Autodesk Inventor part; units mm, degrees
ref_plane "YZ Plane" through (0, 0, 0) normal (1, 0, 0) x (0, 1, 0)
ref_plane "XZ Plane" through (0, 0, 0) normal (0, 1, 0) x (-1, 0, 0)
ref_plane "XY Plane" through (0, 0, 0) normal (0, 0, 1) x (1, 0, 0)
sketch "Szkic1" plane through (0, 0, 0) normal (0, 0, 1) x (1, 0, 0)
  line L0 (-13.054, 5.3954) -> (8.946, 5.3954)
  line L1 (8.946, 5.3954) -> (8.946, -6.6046)
  line L2 (8.946, -6.6046) -> (-13.054, -6.6046)
  line L3 (-13.054, -6.6046) -> (-13.054, 5.3954)
  point P0 (0, 0)
  dimension "d0" = 22
  dimension "d1" = 12
extrude "Wyciągnięcie proste1" add sketch "Szkic1" along normal blind 12.7
fillet "Zaokrąglenie1" radius 2.5 2 edges at (-13.054, 5.3954, 6.35) (8.946, 5.3954, 6.35)
sketch "Szkic2" plane through (0, 0, 12.7) normal (0, 0, 1) x (1, 0, 0)
  line L0 (8.946, -6.6046) -> (8.946, 2.8954)
  line L1 (-13.054, 2.8954) -> (-13.054, -6.6046)
  circle A0 centre (-2.054, -6.8046) radius 8.075
  line L2 (6.446, 5.3954) -> (-10.554, 5.3954)
  point P0 (0, 0)
  dimension "d5" = 22
  dimension "d6" = 11
  dimension "d7" = 16.15
  dimension "d10" = 12.2
extrude "Wyciągnięcie proste2" cut sketch "Szkic2" against normal blind 12.7
sketch "Szkic3" plane through (0, 0, 12.7) normal (0, 0, 1) x (1, 0, 0)
  arc A0 (6.0185, -6.6046) -> (-10.1265, -6.6046) centre (-2.054, -6.8046) ccw
  line L0 (6.0185, -6.6046) -> (8.946, -6.6046)
  line L1 (8.946, -6.6046) -> (8.946, 2.8954)
  arc A1 (8.946, 2.8954) -> (6.446, 5.3954) centre (6.446, 2.8954) ccw
  line L2 (6.446, 5.3954) -> (-10.554, 5.3954)
  arc A2 (-10.554, 5.3954) -> (-13.054, 2.8954) centre (-10.554, 2.8954) ccw
  line L3 (-13.054, 2.8954) -> (-13.054, -6.6046)
  line L4 (-13.054, -6.6046) -> (-10.1265, -6.6046)
  arc A3 (3.9927, -6.6046) -> (-8.1007, -6.6046) centre (-2.054, -6.8046) ccw
  arc A4 (6.0185, -6.6046) -> (-10.1265, -6.6046) centre (-2.054, -6.8046) ccw
  line L5 (6.0185, -6.6046) -> (-10.1265, -6.6046)
  point P0 (0, 0)
  dimension "d11" = 12.1
extrude "Wyciągnięcie proste3" add sketch "Szkic3" against normal blind 8.55 contours L5 A3 A0
extrude "Wyciągnięcie proste4" cut sketch "Szkic3" against normal blind 3.45 contours L5 A3 A0
sketch "Szkic4" plane through (-13.054, -6.6046, 0) normal (0, -1, 0) x (1, 0, 0)
  line L0 (0, 0) -> (0, 12.7)
  line L1 (22, 0) -> (22, 12.7)
  line L2 (4.9533, 9.25) -> (2.9275, 9.25)
  line L3 (19.0725, 9.25) -> (17.0467, 9.25)
  line L4 (4.9533, 9.25) -> (4.9533, 4.15)
  line L5 (4.9533, 4.15) -> (2.9275, 4.15)
  point P0 (13.054, 0)
  point P1 (2.4767, 6.7)
  point P2 (19.5233, 6.7)
  dimension "d16" = 2.4766
  dimension "d17" = 2.4766
  dimension "d18" = 2.55
  dimension "d19" = 2.55
  dimension "d33" = 4.9533
  dimension "d34" = 5.1
hole "Otwór1" at (-10.5773, -6.6046, 6.7) at (6.4694, -6.6046, 6.7) direction (0, 1, 0) diameter 3.2 end through all
sketch "Szkic5" plane through (-10.554, 5.3954, 0) normal (0, 1, 0) x (1, 0, 0)
  arc A0 (0, -8.2998) -> (0, -5.1002) centre (-0.0233, -6.7) ccw
  line L0 (0, -12.7) -> (0, -8.2998)
  line L1 (17, -12.7) -> (0, -12.7)
  line L2 (17, -8.2998) -> (17, -12.7)
  arc A1 (17, -5.1002) -> (17, -8.2998) centre (17.0233, -6.7) ccw
  line L3 (17, 0) -> (17, -5.1002)
  line L4 (0, 0) -> (17, 0)
  line L5 (0, -5.1002) -> (0, 0)
  line L6 (19.5, -12.7) -> (19.5, 0)
  line L7 (-2.5, 0) -> (-2.5, -12.7)
  line L8 (-3.125, -4.9102) -> (-0.025, -3.1204)
  line L9 (-0.025, -3.1204) -> (3.075, -4.9102)
  line L10 (3.075, -4.9102) -> (3.075, -8.4898)
  line L11 (3.075, -8.4898) -> (-0.025, -10.2796)
  line L12 (-0.025, -10.2796) -> (-3.125, -8.4898)
  line L13 (-3.125, -8.4898) -> (-3.125, -4.9102)
  line L14 (13.9, -4.9102) -> (17, -3.1204)
  line L15 (17, -3.1204) -> (20.1, -4.9102)
  line L16 (20.1, -4.9102) -> (20.1, -8.4898)
  line L17 (20.1, -8.4898) -> (17, -10.2796)
  line L18 (17, -10.2796) -> (13.9, -8.4898)
  line L19 (13.9, -8.4898) -> (13.9, -4.9102)
  point P0 (10.554, 0)
  point P1 (17, -6.7)
  point P2 (-0.025, -6.7)
  point P3 (-0.025, -6.7)
  point P4 (-3.125, -6.7)
  point P5 (17, -6.7)
  point P6 (13.9, -6.7)
extrude "Wyciągnięcie proste6" cut sketch "Szkic5" against normal blind 4 contours L0 L11 L12 L7 L8 L9 L5 A0 | A0 L5 L9 L10 L11 L0 | L12 L13 L8 L7 | L18 L19 L14 L3 A1 L2 | L2 A1 L3 L15 L6 L17 | L6 L15 L16 L17
properties part number "3DP_ABS_E3DV6_Mounting_Clamp"
Here's how the part is built. I have some questions about the finished solid (model axes, mm). A direction names the side the tool comes from. Give positions to 0.01 mm unless a question says otherwise; leave off trailing zeros. Loops run counter-clockwise (first coordinate to the right, second up) from the corner with the lowest first, then second, coordinate; pieces in that order, holes last. Notation, with made-up numbers: M -4.5,16.5 L 51.5,16.5 A25 ccw 51.5,35.5 Z; hole C 43,68.5 d8. An arc over 180 degrees is marked long. Return JSON: item names as keys, results as strings.
Item 1: Imagine slicing it at D-D on y = 2.5. List the corners of the cut face in (x, z) for me.
A:
{"outline": "M -13.05,0 L 8.95,0 L 8.95,4.56 L 6.45,3.12 L 3.35,4.91 L 3.35,8.49 L 6.45,10.28 L 8.95,8.84 L 8.95,12.7 L -13.05,12.7 L -13.05,8.85 L -10.58,10.28 L -7.48,8.49 L -7.48,4.91 L -10.58,3.12 L -13.05,4.55 Z"}
Item 2: I'm going to push flat-ended pins straight in: pin 1 Ø6 at (x, z) = (7, 7) entering from +Y; pin 2 Ø1.5 at (x, y) = (3, -4.5) entering from -Z; pin 3 Ø5 at (y, z) = (3, 6) entering from +X; pin 4 Ø1.1 at (y, z) = (3, 7) entering from +X. Where does each tip first touch, or does it pass through?
A:
{"pin 1": "stops at y = 5.35", "pin 2": "stops at z = 4.15", "pin 3": "stops at x = 8.95", "pin 4": "stops at x = 3.35"}
Item 3: Please list where these lines run through material, in increasing order: line 1 (X direction, y = -3, z = 6.7); line 2 (X direction, y = -3.75, z = 6.7); line 3 (X direction, y = -3.75, z = 9.5).
A:
{"line 1": "x = -13.05 to -12.18, -8.98 to -6.76, 2.65 to 4.87, 8.07 to 8.95", "line 2": "x = -13.05 to -12.18, -8.98 to -7.28, 3.17 to 4.87, 8.07 to 8.95", "line 3": "x = -13.05 to -9.53, 5.42 to 8.95"}
Item 4: Imagine slicing it at A-A on z = 6.7. List the corners of the cut face in (x, y) for me.
A:
{"outline": "M -13.05,-6.6 L -12.18,-6.6 L -12.18,1.4 L -13.05,1.4 Z; M -8.98,-6.6 L -8.1,-6.6 A6.05 cw 3.99,-6.6 L 4.87,-6.6 L 4.87,1.4 L 3.35,1.4 L 3.35,5.4 L -7.48,5.4 L -7.48,1.4 L -8.98,1.4 Z; M 8.07,-6.6 L 8.95,-6.6 L 8.95,1.4 L 8.07,1.4 Z"}
Item 5: Imagine slicing it at C-C on x = 7. List the corners of the cut face in (y, z) for me, then the cut area to 3 significant figures.
A:
{"outline": "M -6.6,0 L 5.33,0 L 5.33,3.44 L 1.4,3.44 L 1.4,5.19 L -6.6,5.19 Z; M -6.6,8.21 L 1.4,8.21 L 1.4,9.96 L 5.33,9.96 L 5.33,12.7 L -6.6,12.7 Z", "area": "102 mm^2"}
Item 6: Imagine slicing it at B-B on y = -2.25. List the corners of the cut face in (x, z) for me.
A:
{"outline": "M -13.05,0 L -8.72,0 L -8.72,4.15 L -6.04,4.15 L -6.04,9.25 L -8.72,9.25 L -8.72,12.7 L -13.05,12.7 Z; M 1.93,4.15 L 4.61,4.15 L 4.61,0 L 8.95,0 L 8.95,12.7 L 4.61,12.7 L 4.61,9.25 L 1.93,9.25 Z; hole C -10.58,6.7 d3.2; hole C 6.47,6.7 d3.2"}
Item 7: Thinking about a two-plate mould opening in Z: for faces 1 (the flat face through (-2, 5.395, 6)), 2 (the flat face through (4.9, 1.395, 5.9)), 3 (the flat face through (-2, 2, 0)), which applies, released by +Z, released by -Z, zero draft, split by the parting line, or undercut?
A:
{"face 1": "zero draft", "face 2": "undercut", "face 3": "released by -Z"}
Item 8: On a 3-axis mill with a long thin cutter (end or side, diameter ignored), from which of +Z, -Z, +X, -X, +Y, -Y can I reach the whole of each face in a straight line? I mean faces 4 (the flat face through (3.346, 3, 7)), 5 (the cylindrical face through (8.233, 4.644, 10.795)), 6 (the flat face through (-11.834, 2.979, 3.845)), 7 (the cylindrical face through (-1.88, 1.27, 2.1)). Say none if no direction works.
A:
{"face 4": "+X, +Y", "face 5": "+Z, -Z, +X, +Y", "face 6": "+Y", "face 7": "-Z, -Y"}
